```python
from build123d import *

# Parameters (mm, degrees)
SKETCH_1_R          = 2
SKETCH_1_R_2        = 6.4
EXTRUDE_1_DEPTH     = 2.5
EXTRUDE_START       = 2
SKETCH_2_R          = 10.5
SKETCH_2_R_2        = 6.4
EXTRUDE_2_DEPTH     = 2
SKETCH_3_R          = 11
CUT_EXTRUDE_1_DEPTH = 1
SKETCH_4_R          = 7
SKETCH_4_R_2        = 6.4
EXTRUDE_3_DEPTH     = 42
FILLET_2_R          = 1
SKETCH_5_R          = 7
SKETCH_5_R_2        = 4
EXTRUDE_4_DEPTH     = 1.5
FILLET_3_R          = 5
FILLET_4_R          = 2


with BuildPart() as part:
    # 草图1 → 凸台-拉伸1 (new body)
    with BuildSketch(Plane(origin=(0, 0, 0), x_dir=(1, 0, 0), z_dir=(0, 1, 0))):
        with BuildLine():
            ThreePointArc((3, 26), (0, 35), (-3, 26))
            Line((-3, 26), (-3, 14.696938457))
            ThreePointArc((-3, 14.696938457), (-12.990381057, 7.5), (-14.227922061, -4.750393017))
            Line((-14.227922061, -4.750393017), (-24.016660498, -10.401923789))
            ThreePointArc((-24.016660498, -10.401923789), (-30.310889132, -17.5), (-21.016660498, -15.598076211))
            Line((-21.016660498, -15.598076211), (-11.227922061, -9.94654544))
            ThreePointArc((-11.227922061, -9.94654544), (0, -15), (11.227922061, -9.94654544))
            Line((11.227922061, -9.94654544), (21.016660498, -15.598076211))
            ThreePointArc((21.016660498, -15.598076211), (30.310889132, -17.5), (24.016660498, -10.401923789))
            Line((24.016660498, -10.401923789), (14.227922061, -4.750393017))
            ThreePointArc((14.227922061, -4.750393017), (12.990381057, 7.5), (3, 14.696938457))
            Line((3, 14.696938457), (3, 26))
        make_face()
        with Locations(Location((-25.980762114, -15, 0), (0, 0, 270))):
            Circle(SKETCH_1_R, mode=Mode.SUBTRACT)
        with Locations(Location((0, 0, 0), (0, 0, 270))):
            Circle(SKETCH_1_R_2, mode=Mode.SUBTRACT)
        with Locations(Location((0, 30, 0), (0, 0, 270))):
            Circle(SKETCH_1_R, mode=Mode.SUBTRACT)
        with Locations(Location((25.980762114, -15, 0), (0, 0, 270))):
            Circle(SKETCH_1_R, mode=Mode.SUBTRACT)
    extrude(amount=-EXTRUDE_1_DEPTH)

    # 草图2 → 凸台-拉伸2 (add)
    with BuildSketch(Plane(origin=(0, 0, 0), x_dir=(1, 0, 0), z_dir=(0, 1, 0)).offset(EXTRUDE_START)):
        with Locations(Location((0, 0, 0), (0, 0, 270))):
            Circle(SKETCH_2_R)
        with Locations(Location((0, 0, 0), (0, 0, 270))):
            Circle(SKETCH_2_R_2, mode=Mode.SUBTRACT)
    extrude(amount=-EXTRUDE_2_DEPTH)

    # 草图3 → 切除-拉伸1 (cut)
    with BuildSketch(Plane.XZ.offset(2.5)):
        with Locations(Location((0, 0, 0), (0, 0, 270))):
            Circle(SKETCH_3_R)
    extrude(amount=-CUT_EXTRUDE_1_DEPTH, mode=Mode.SUBTRACT)

    # 草图4 → 凸台-拉伸3 (add)
    with BuildSketch(Plane.XZ.offset(1.5)):
        with Locations(Location((0, 0, 0), (0, 0, 90))):
            Circle(SKETCH_4_R)
        with Locations(Location((0, 0, 0), (0, 0, 90))):
            Circle(SKETCH_4_R_2, mode=Mode.SUBTRACT)
    extrude(amount=EXTRUDE_3_DEPTH)

    # 圆角2
    fillet_2_edges = [part.edges().sort_by_distance(p)[0] for p in [
        (0, 2, -6.4),
        (0, -1.5, -7),
    ]]
    fillet(fillet_2_edges, radius=FILLET_2_R)

    # 草图5 → 凸台-拉伸4 (add)
    with BuildSketch(Plane.XZ.offset(43.5)):
        with Locations(Location((0, 0, 0), (0, 0, 90))):
            Circle(SKETCH_5_R)
        with Locations(Location((0, 0, 0), (0, 0, 270))):
            Circle(SKETCH_5_R_2, mode=Mode.SUBTRACT)
    extrude(amount=EXTRUDE_4_DEPTH)

    # 圆角3
    fillet_3_edges = [part.edges().sort_by_distance(p)[0] for p in [
        (-24.016660498, -1.25, 10.401923789),
        (-14.227922061, -1.25, 4.750393017),
        (-3, -1.25, -14.696938457),
        (-3, -1.25, -26),
        (3, -1.25, -26),
        (3, -1.25, -14.696938457),
        (14.227922061, -1.25, 4.750393017),
        (24.016660498, -1.25, 10.401923789),
        (21.016660498, -1.25, 15.598076211),
        (11.227922061, -1.25, 9.94654544),
        (-11.227922061, -1.25, 9.94654544),
        (-21.016660498, -1.25, 15.598076211),
    ]]
    fillet(fillet_3_edges, radius=FILLET_3_R)

    # 圆角4
    fillet_4_edges = [part.edges().sort_by_distance(p)[0] for p in [
        (0, 0, -10.5),
    ]]
    fillet(fillet_4_edges, radius=FILLET_4_R - 0.0001)  # a hair under: the kernel refuses the full size


solid = part.part
```
Check sheet for the modelled part. Datum: model origin and axes. Units: mm. A direction names the side the tool comes from. Round coordinates to 2 decimals unless told otherwise and drop trailing zeros. Order: outer loops, then holes, each group sorted by start corner. A loop starts at its lowest first (then second) coordinate and runs counter-clockwise, first axis right, second up.
1) Section check D-D (y = -28). Record the boundary of the cut face in (x, z), and give its area (3 significant figures).
2) Mould release check, pull along X, two halves, no side actions. Record for faces 1 (the cylindrical face through (-3.84, -1.27, -15.56)), 2 (the cylindrical face through (15.43, -1.27, 4.53)), 3 (the cylindrical face through (11.6, -1.3, 11.1)): +X half, -X half, draft (parallel to the pull), parting line (faces both ways), or undercut.
3) Section check A-A (z = -30). Record the boundary of the cut face in (x, y).
4) Scan lines: line 1 (X direction, y = -1, z = 0); line 2 (X direction, y = -1.7, z = 0); line 3 (X direction, y = -8, z = 0). Record each from-to range of solid material in increasing order.
5) Section check B-B (x = 0). Give the number of separate pieces and of enclosed holes in the cut face, and give its area (3 significant figures).
6) Tool access check on faces 4 (the flat face through (-16.86, -1.23, 13.2)), 5 (the cylindrical face through (-10.74, -2.01, 2.38)), 6 (the flat face through (-3, -1, -21)), 7 (the flat face through (-9, 0, 9)), 8 (the cylindrical face through (3.84, -1.27, -15.56)). Record the directions out of +Z, -Z, +X, -X, +Y, -Y that give a thin tool (end or side, any length) a straight path to the whole face; none if there is none.
7) Go/stop test with flat-tipped pins: pin 1 Ø4.5 at (x, z) = (-25.98, 15) entering from -Y; pin 2 Ø4 at (x, y) = (-10, -31) entering from +Z; pin 3 Ø0.8 at (y, z) = (-1, -20.5) entering from +X; pin 4 Ø12 at (x, z) = (-19.5, -4.5) entering from +Y. Record where each tip stops, or that it passes through.
Result:
1. outline: circle Ø14 at (0, 0); hole circle Ø12.8 at (0, 0)
1. area: 25.3 mm2
2. face 1: -X half
2. face 2: +X half
2. face 3: undercut
3. outline: (-5, -2.5) - (-2, -2.5) - (-2, 0) - (-5, 0) - close; (2, -2.5) - (5, -2.5) - (5, 0) - (2, 0) - close
4. line 1: x = -15 to -6.4, 6.4 to 15
4. line 2: x = -15 to -11, -7.4 to -6.4, 6.4 to 7.4, 11 to 15
4. line 3: x = -7 to -6.4, 6.4 to 7
5. separate pieces: 3
5. enclosed holes: 0
5. area: 151 mm2
6. face 4: +Z, +Y, -Y
6. face 5: -Y
6. face 6: -X, +Y, -Y
6. face 7: +Y
6. face 8: +X, +Y, -Y
7. pin 1: stops at y = -2.5
7. pin 2: passes through
7. pin 3: stops at x = 3
7. pin 4: stops at y = 0
